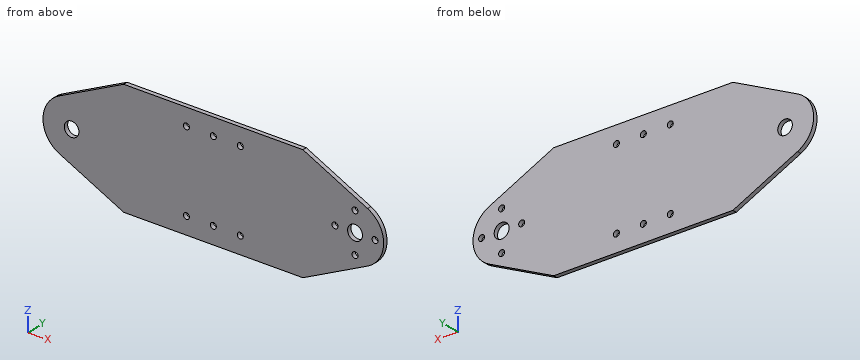
Autodesk Inventor part; units mm, degrees
ref_plane "YZ Plane" through (0, 0, 0) normal (1, 0, 0) x (0, 1, 0)
ref_plane "XZ Plane" through (0, 0, 0) normal (0, 1, 0) x (-1, 0, 0)
ref_plane "XY Plane" through (0, 0, 0) normal (0, 0, 1) x (1, 0, 0)
sketch "Sketch1" plane through (0, 0, 0) normal (0, 1, 0) x (-1, 0, 0)
  line L0 (-32.1589, 0) -> (-32.1589, -40)
  line L1 (-0.4496, -40) -> (-0.4496, 0)
  circle A0 centre (-72.7986, -20) radius 1.05
  circle A1 centre (-65.7986, -13) radius 1.05
  circle A2 centre (-65.7986, -27) radius 1.05
  circle A3 centre (-58.7986, -20) radius 1.05
  circle A4 centre (-25.7093, -6) radius 1.05
  circle A5 centre (-25.7093, -34) radius 1.05
  circle A6 centre (-16.3043, -6) radius 1.05
  circle A7 centre (-16.3043, -34) radius 1.05
  circle A8 centre (-6.8993, -6) radius 1.05
  circle A9 centre (-6.8993, -34) radius 1.05
  circle A10 centre (-65.7986, -20) radius 2.6
  circle A11 centre (33.19, -20) radius 2.55
  line L2 (37.5744, -11.0124) -> (15, 0)
  arc A12 (37.5744, -28.9876) -> (37.5744, -11.0124) centre (33.19, -20) ccw
  line L3 (15, -40) -> (37.5744, -28.9876)
  line L4 (-47.6086, 0) -> (-70.183, -11.0124)
  arc A13 (-70.183, -11.0124) -> (-70.183, -28.9876) centre (-65.7986, -20) ccw
  line L5 (-70.183, -28.9876) -> (-47.6086, -40)
  line L6 (-47.6086, 0) -> (15, 0)
  line L7 (15, -40) -> (-47.6086, -40)
  line L8 (-32.6086, -40) -> (-32.6086, 0)
  line L9 (-31.7093, 0) -> (-31.7093, -40)
  line L10 (-0.8993, -40) -> (-0.8993, 0)
  line L11 (0, 0) -> (0, -40)
extrude "Extrusion1" add sketch "Sketch1" against normal blind 1.5
properties part number "CAM_axis_6_bottom_frame(top)"
Can you work these out from the model? Positions are in its coordinate system, mm. Coordinates: 2 decimals unless noted, no trailing zeros. Loops run counter-clockwise (first coordinate to the right, second up) from the corner with the lowest first, then second, coordinate; pieces in that order, holes last.
1) Imagine slicing it at C-C on z = -13. List the corners of the cut face in (x, y) for me, plus the area to 3 significant figures.
2) Imagine slicing it at D-D on x = -33.19. List the corners of the cut face in (y, z) for me.
3) I need wall thicknesses on probe 1 along Z at (x, y) = (25, -0.15); probe 2 along Z at (x, y) = (7.5, -0.9); probe 3 along X at (y, z) = (-0.9, -6.5). Which ranges of each line are inside material? Lowest first, please.
4) Imagine slicing it at B-B on y = -0.4. State how many separate pieces and enclosed holes the cut face has, plus the area to 3 significant figures.
5) Imagine slicing it at A-A on z = -20. List the corners of the cut face in (x, y) for me, plus the area to 3 significant figures.
6) For pin 1 (1.7 mm diameter, centred on x = 6.9, z = -6, fed in from -Y), with a flat end and sliding along its axis, tell me the tip position at first contact or that it passes through.
Completed:
1. outline: (-40.33, -1.5) - (64.75, -1.5) - (64.75, 0) - (-40.33, 0) - close; (66.85, -1.5) - (72.94, -1.5) - (72.94, 0) - (66.85, 0) - close
1. area: 167 mm2
2. outline: (-1.5, -31.13) - (0, -31.13) - (0, -22.55) - (-1.5, -22.55) - close; (-1.5, -17.45) - (0, -17.45) - (0, -8.87) - (-1.5, -8.87) - close
3. probe 1: z = -40 to -34.77, -33.23 to -6.77, -5.23 to 0
3. probe 2: z = -40 to -34.86, -33.14 to -6.86, -5.14 to 0
3. probe 3: x = -28.32 to 5.98, 7.82 to 15.38, 17.23 to 24.79, 26.63 to 60.93
4. separate pieces: 1
4. enclosed holes: 12
4. area: 3,880 mm2
5. outline: (-43.19, -1.5) - (-35.74, -1.5) - (-35.74, 0) - (-43.19, 0) - close; (-30.64, -1.5) - (57.75, -1.5) - (57.75, 0) - (-30.64, 0) - close; (59.85, -1.5) - (63.2, -1.5) - (63.2, 0) - (59.85, 0) - close; (68.4, -1.5) - (71.75, -1.5) - (71.75, 0) - (68.4, 0) - close; (73.85, -1.5) - (75.8, -1.5) - (75.8, 0) - (73.85, 0) - close
5. area: 157 mm2
6. pin 1: passes through
